Source: CAD feature listing. Evaluate the final solid. Frame: model axes, mm. Give positions to 0.01 mm unless a question says otherwise; leave off trailing zeros. Order: outer loops, then holes, each group sorted by start corner. A loop starts at its lowest first (then second) coordinate and runs counter-clockwise, first axis right, second up.
```python
from build123d import *

# Parameters (mm, degrees)
F0_W     = 241.3
F0_H     = 101.6
F1_DEPTH = 6.35
F2_W     = 76.2
F2_H     = 6.35
F3_DEPTH = 6.35
F4_W     = 6.35
F4_H     = 50.8
F5_DEPTH = 6.35


with BuildPart() as f1:
    # F0 (on Front) → F1 (new body)
    with BuildSketch(Plane.XZ):
        with Locations((0, 50.8)):
            Rectangle(F0_W, F0_H)
    extrude(amount=F1_DEPTH)

    # F2 (on face) → F3 (join)
    with BuildSketch(Plane.XZ.offset(6.35)):
        with Locations((0, -3.175)):
            Rectangle(F2_W, F2_H)
    extrude(amount=-F3_DEPTH)

    # F4 (on face) → F5 (join)
    with BuildSketch(Plane.XZ.offset(6.35)):
        with Locations((-123.825, 50.8)):
            Rectangle(F4_W, F4_H)
        with Locations((123.825, 50.8)):
            Rectangle(F4_W, F4_H)
    extrude(amount=-F5_DEPTH)


solid = f1.part
```
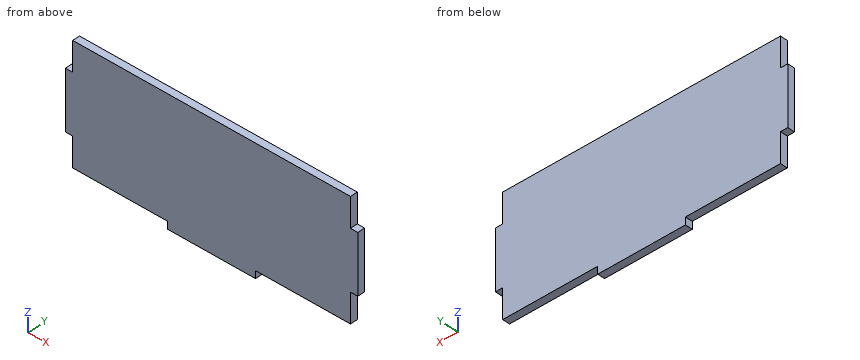
1) Section query B-B, the plane z = 20.5. Return the cut outline in (x, y), and give its area (3 significant figures).
Report:
outline: (-120.65, -6.35) - (120.65, -6.35) - (120.65, 0) - (-120.65, 0) - close
area: 1,530 mm2
2) Section query C-C, the plane x = -111. Return the cut outline in (y, z), and give its area (3 significant figures).
Report:
outline: (-6.35, 0) - (0, 0) - (0, 101.6) - (-6.35, 101.6) - close
area: 645 mm2
3) Material intervals for L1, parallel to Z at x = 83, y = -2; L2, parallel to X at y = -0.75, z = 15, sorted ascending.
Report:
L1: z = 0 to 101.6
L2: x = -120.65 to 120.65
4) Section query A-A, the plane y = -3.25. Return the cut outline in (x, z).
Report:
outline: (-127, 25.4) - (-120.65, 25.4) - (-120.65, 0) - (-38.1, 0) - (-38.1, -6.35) - (38.1, -6.35) - (38.1, 0) - (120.65, 0) - (120.65, 25.4) - (127, 25.4) - (127, 76.2) - (120.65, 76.2) - (120.65, 101.6) - (-120.65, 101.6) - (-120.65, 76.2) - (-127, 76.2) - close
5) Pin query (flat end, axial travel): pin 1 (3 mm diameter, centred on y = -2.5, z = 86.5, fed in from -X); pin 2 (1.9 mm diameter, centred on x = -61, y = -3.5, fed in from -Z); pin 3 (1.9 mm diameter, centred on y = -3.5, z = -2, fed in from -X). Return the tip coordinate at first contact, or that it passes through.
Report:
pin 1: stops at x = -120.65
pin 2: stops at z = 0
pin 3: stops at x = -38.1
